Geometry check sheet. Reference: the model listing, model coordinates, mm. Coordinates: 2 decimals unless noted, no trailing zeros. Order: outer loops, then holes, each group sorted by start corner. A loop starts at its lowest first (then second) coordinate and runs counter-clockwise, first axis right, second up. Notation, with made-up numbers: M -19.5,22.25 L 29.5,22.25 A18 cw 29.5,44.25 Z; hole C 71.25,78.5 d9. An arc over 180 degrees is marked long. One line per item, written item: value. Start each with the question number.
1) Sectioned sample at C-C, the plane y = 4.25. Enter the section's corners in (x, z).
2) Sectioned sample at B-B, the plane z = 130. Enter the section's corners in (x, y).
3) Draft check along Z on faces 1 (the flat face through (0, 0, 190)), 2 (the cylindrical face through (-0.14, 0.46, 127.95)), 3 (the flat face through (0, 0, 0)), 4 (the flat face through (-10, 0, 94)). Enter one of: pulls with the +Z half, pulls with the -Z half, needs draft (parallel to the pull), parting line crosses it, or undercut.
4) Thickness scan on L1, parallel to Y at x = -1.5, z = 170; L2, parallel to X at y = -9, z = 179.5. Record the ranges inside material, lowest first. Write a range as from..to.
5) Sectioned sample at A-A, the plane x = 0. State how many separate pieces and enclosed holes the cut face has, then the cut area to 3 significant figures.
```python
from build123d import *

# Parameters (mm, degrees)
SKETCH_1_W          = 20
SKETCH_1_H          = 20
EXTRUDE_1_DEPTH     = 190
SKETCH_2_R          = 2.1
CUT_EXTRUDE_1_DEPTH = 67
SKETCH_3_R          = 2.1
CUT_EXTRUDE_2_DEPTH = 32
SKETCH_4_R          = 2.1
CUT_EXTRUDE_3_DEPTH = 192.311264697


with BuildPart() as part:
    # 草图1 → 凸台-拉伸1 (new body)
    with BuildSketch(Plane.XY):
        Rectangle(SKETCH_1_W, SKETCH_1_H)
    extrude(amount=EXTRUDE_1_DEPTH)

    # 草图2 → 切除-拉伸1 (cut)
    with BuildSketch(Plane.ZY.offset(10)):
        with Locations(Location((40, 0, 0), (0, 0, 270))):
            Circle(SKETCH_2_R)
        with Locations(Location((20, 0, 0), (0, 0, 270))):
            Circle(SKETCH_2_R)
        with Locations(Location((60, 0, 0), (0, 0, 270))):
            Circle(SKETCH_2_R)
        with Locations(Location((130, 0, 0), (0, 0, 270))):
            Circle(SKETCH_2_R)
        with Locations(Location((170, 0, 0), (0, 0, 270))):
            Circle(SKETCH_2_R)
        with Locations(Location((150, 0, 0), (0, 0, 270))):
            Circle(SKETCH_2_R)
    extrude(amount=-CUT_EXTRUDE_1_DEPTH, mode=Mode.SUBTRACT)

    # 草图3 → 切除-拉伸2 (cut)
    with BuildSketch(Plane(origin=(0, 10, 0), x_dir=(1, 0, 0), z_dir=(0, 1, 0))):
        with Locations(Location((0, -180, 0), (0, 0, 270))):
            Circle(SKETCH_3_R)
        with Locations(Location((0, -165, 0), (0, 0, 270))):
            Circle(SKETCH_3_R)
        with Locations(Location((0, -25, 0), (0, 0, 270))):
            Circle(SKETCH_3_R)
        with Locations(Location((0, -10, 0), (0, 0, 270))):
            Circle(SKETCH_3_R)
    extrude(amount=-CUT_EXTRUDE_2_DEPTH, mode=Mode.SUBTRACT)

    # 草图4 → 切除-拉伸3 (cut, through all)
    with BuildSketch(Plane(origin=(0, 10, 0), x_dir=(1, 0, 0), z_dir=(0, 1, 0))):
        with Locations(Location((0, -85, 0), (0, 0, 270))):
            Circle(SKETCH_4_R)
        with Locations(Location((0, -105, 0), (0, 0, 90))):
            Circle(SKETCH_4_R)
    extrude(amount=-CUT_EXTRUDE_3_DEPTH, mode=Mode.SUBTRACT)


solid = part.part
```
Final values:
1. outline: M -10,0 L 10,0 L 10,190 L -10,190 Z; hole C 0,10 d4.2; hole C 0,25 d4.2; hole C 0,85 d4.2; hole C 0,105 d4.2; hole C 0,165 d4.2; hole C 0,180 d4.2
2. outline: M -10,-10 L 10,-10 L 10,-2.1 L -10,-2.1 Z; M -10,2.1 L 10,2.1 L 10,10 L -10,10 Z
3. face 1: pulls with the +Z half
3. face 2: undercut
3. face 3: pulls with the -Z half
3. face 4: needs draft
4. L1: y = -10..-2.1, 2.1..10
4. L2: x = -10..-2.04, 2.04..10
5. separate pieces: 7
5. enclosed holes: 6
5. area: 3,210 mm^2
